Autodesk Inventor part; units mm, degrees
ref_plane "YZ Plane" through (0, 0, 0) normal (1, 0, 0) x (0, 1, 0)
ref_plane "XZ Plane" through (0, 0, 0) normal (0, 1, 0) x (-1, 0, 0)
ref_plane "XY Plane" through (0, 0, 0) normal (0, 0, 1) x (1, 0, 0)
sketch "Sketch1" plane through (0, 0, 0) normal (0, 1, 0) x (-1, 0, 0)
  line L0 (10.2019, 0) -> (-11.9707, 0)
  line L1 (0, 17.6887) -> (0, -16.1667)
  line L2 (250, 300) -> (-250, 300)
  line L3 (-250, 300) -> (-250, -300)
  line L4 (-250, -300) -> (250, -300)
  line L5 (250, -300) -> (250, 300)
  point P0 (0, 0)
  dimension "d0" = 600
  dimension "d1" = 500
extrude "Extrusion1" add sketch "Sketch1" along normal blind 10
sketch "Sketch2" plane through (-250, 0, 300) normal (0, 0, 1) x (1, 0, 0)
  line L0 (0, 0) -> (500, 0)
  line L1 (500, 0) -> (500, 300)
  line L2 (500, 300) -> (0, 300)
  line L3 (0, 300) -> (0, 0)
  point P0 (250, 0)
  dimension "d4" = 300
  dimension "d5" = 500
extrude "Extrusion2" add sketch "Sketch2" along normal blind 10
properties part number "ground"
For this review, take the finished solid that the model builds, in its own axes (mm). A direction names the side the tool comes from. Coordinates: 2 decimals unless noted, no trailing zeros. Write each loop counter-clockwise with the first axis right and the second up, starting at its lowest first coordinate (ties: lowest second). Pieces come first, ordered by that corner, then holes.
(1) Add section A-A on x = 204. Give the boundary of the cut face in (y, z).
(2) Tool access review of faces 1 (the face through (-3, 152, 310)), 2 (the face through (-3, 157, 300)): name each direction out of +Z, -Z, +X, -X, +Y, -Y from which nothing blocks a thin tool from reaching the whole face with its end or side.
(3) Add section C-C on z = -261. Give the boundary of the cut face in (x, y), then the cut area to 3 significant figures.
(4) For pin 1 Ø12 at (x, z) = (123.5, -34) entering from +Y; pin 2 Ø2 at (x, y) = (-98.5, 64) entering from -Z, all flat-tipped, find the tip position at first contact; note any pin that passes through.
(5) Wall thickness on probe 1 along Z at (x, y) = (-150.5, 284); probe 2 along Y at (x, z) = (120.5, 110): over which ranges is each line inside the solid? List them lowest first.
(6) Add section B-B on y = 277.5. Give the boundary of the cut face in (x, z), then the cut area to 3 significant figures.
Answer sheet:
1. outline: (0, -300) - (10, -300) - (10, 300) - (300, 300) - (300, 310) - (0, 310) - close
2. face 1: +Z, +X, -X, +Y, -Y
2. face 2: -Z, +X, -X, +Y
3. outline: (-250, 0) - (250, 0) - (250, 10) - (-250, 10) - close
3. area: 5,000 mm2
4. pin 1: stops at y = 10
4. pin 2: stops at z = 300
5. probe 1: z = 300 to 310
5. probe 2: y = 0 to 10
6. outline: (-250, 300) - (250, 300) - (250, 310) - (-250, 310) - close
6. area: 5,000 mm2
